from build123d import *

# Parameters (mm, degrees)
SKETCH1_R             = 0.6
BOSS_EXTRUDE1_DEPTH   = 1
SKETCH1_W             = 37.4
SKETCH1_H             = 2.5
BOSS_EXTRUDE1_2_DEPTH = 1
BOSS_EXTRUDE1_3_DEPTH = 1
BOSS_EXTRUDE1_4_DEPTH = 1
SKETCH1_W_2           = 9.2
BOSS_EXTRUDE1_5_DEPTH = 1
BOSS_EXTRUDE2_DEPTH   = 1.5
SKETCH4_W             = 3.5
SKETCH4_H             = 2.5
BOSS_EXTRUDE3_DEPTH   = 3.8
FILLET1_R             = 0.4


with BuildPart() as part:
    # Sketch1 → Boss-Extrude1 (new body)
    with BuildSketch(Plane(origin=(0, 0, 0), x_dir=(1, 0, 0), z_dir=(0, 1, 0))):
        Polygon((-22.2, 30), (-25.229966902, 30), (-40, 30), (-40, 0), (-25.229966902, 0), (-22.2, 0), (-22.2, 2.5), (-37.5, 2.5), (-37.5, 27.5), (-22.2, 27.5), align=None)
        with Locations((-38.75, 1.25)):
            Circle(SKETCH1_R, mode=Mode.SUBTRACT)
        with Locations((-38.75, 28.75)):
            Circle(SKETCH1_R, mode=Mode.SUBTRACT)
    extrude(amount=-BOSS_EXTRUDE1_DEPTH)



with BuildPart() as body_2:
    # Sketch1 → Boss-Extrude1 2 (new body)
    with BuildSketch(Plane(origin=(0, 0, 0), x_dir=(1, 0, 0), z_dir=(0, 1, 0))):
        with Locations((0, 1.25)):
            Rectangle(SKETCH1_W, SKETCH1_H)
    extrude(amount=-BOSS_EXTRUDE1_2_DEPTH)


with BuildPart() as body_3:
    # Sketch1 → Boss-Extrude1 3 (new body)
    with BuildSketch(Plane(origin=(0, 0, 0), x_dir=(1, 0, 0), z_dir=(0, 1, 0))):
        Polygon((12, 30), (10, 30), (9.5, 30), (9.5, 27.5), (18.7, 27.5), (18.7, 30), align=None)
    extrude(amount=-BOSS_EXTRUDE1_3_DEPTH)


with BuildPart() as body_4:
    # Sketch1 → Boss-Extrude1 4 (new body)
    with BuildSketch(Plane(origin=(0, 0, 0), x_dir=(1, 0, 0), z_dir=(0, 1, 0))):
        Polygon((25.229966902, 30), (22.2, 30), (22.2, 27.5), (37.5, 27.5), (37.5, 2.5), (22.2, 2.5), (22.2, 0), (25.229966902, 0), (40, 0), (40, 30), align=None)
        with Locations((38.75, 1.25)):
            Circle(SKETCH1_R, mode=Mode.SUBTRACT)
        with Locations((38.75, 28.75)):
            Circle(SKETCH1_R, mode=Mode.SUBTRACT)
    extrude(amount=-BOSS_EXTRUDE1_4_DEPTH)


with BuildPart() as body_5:
    # Sketch1 → Boss-Extrude1 5 (new body)
    with BuildSketch(Plane(origin=(0, 0, 0), x_dir=(1, 0, 0), z_dir=(0, 1, 0))):
        with Locations((-14.1, 28.75)):
            Rectangle(SKETCH1_W_2, SKETCH1_H)
    extrude(amount=-BOSS_EXTRUDE1_5_DEPTH)


with BuildPart() as part_1:
    add(part.part)

    add(body_2.part)  # Boss-Extrude2 merges body 2

    add(body_3.part)  # Boss-Extrude2 merges body 3

    add(body_4.part)  # Boss-Extrude2 merges body 4

    add(body_5.part)  # Boss-Extrude2 merges body 5
    # Sketch3 → Boss-Extrude2 (add)
    with BuildSketch(Plane(origin=(0, 0, 0), x_dir=(1, 0, 0), z_dir=(0, 1, 0))):
        Polygon((-22.2, 27.5), (-37.5, 27.5), (-37.5, 2.5), (-22.2, 2.5), (-22.2, 0), (-18.7, 0), (-18.7, 2.5), (-9.5, 2.5), (-9.5, 27.5), (-18.7, 27.5), (-18.7, 30), (-22.2, 30), align=None)
        Polygon((9.5, 27.5), (18.7, 27.5), (18.7, 30), (22.2, 30), (22.2, 27.5), (37.5, 27.5), (37.5, 2.5), (22.2, 2.5), (22.2, 0), (18.7, 0), (18.7, 2.5), (9.5, 2.5), align=None)
    extrude(amount=-BOSS_EXTRUDE2_DEPTH)

    # Sketch4 → Boss-Extrude3 (add)
    with BuildSketch(Plane(origin=(0, 0, 0), x_dir=(1, 0, 0), z_dir=(0, 1, 0))):
        with Locations((-20.45, 28.75)):
            Rectangle(SKETCH4_W, SKETCH4_H)
        with Locations((20.45, 28.75)):
            Rectangle(SKETCH4_W, SKETCH4_H)
        with Locations((-20.45, 1.25)):
            Rectangle(SKETCH4_W, SKETCH4_H)
        with Locations((20.45, 1.25)):
            Rectangle(SKETCH4_W, SKETCH4_H)
    extrude(amount=-BOSS_EXTRUDE3_DEPTH)

    # Fillet1
    fillet1_edges = [part_1.edges().sort_by_distance(p)[0] for p in [
        (-22.2, -2.65, -27.5),
        (-18.7, -2.65, -27.5),
        (-18.7, -2.4, -30),
        (-22.2, -2.4, -30),
        (14.1, -1, -30),
        (18.7, -2.4, -30),
        (20.45, -3.8, -30),
        (22.2, -2.4, -30),
        (31.1, -1, -30),
        (40, -0.5, -30),
        (24.75, 0, -30),
        (9.5, -0.5, -30),
        (-18.7, -2.4, 0),
        (-20.45, -3.8, 0),
        (-22.2, -2.4, 0),
        (-31.1, -1, 0),
        (-40, -0.5, 0),
        (0, 0, 0),
        (40, -0.5, 0),
        (31.1, -1, 0),
        (22.2, -2.4, 0),
        (20.45, -3.8, 0),
        (18.7, -2.4, 0),
        (0, -1, 0),
        (-40, -1, -15),
        (0, -1, -2.5),
        (9.5, -1.5, -15),
        (-9.5, -1.5, -15),
        (40, -1, -15),
        (37.5, -1.5, -15),
        (-37.5, -1.5, -15),
        (-18.7, -2.65, -2.5),
        (-22.2, -2.65, -2.5),
        (18.7, -2.65, -2.5),
        (22.2, -2.65, -2.5),
        (22.2, -2.65, -27.5),
        (18.7, -2.65, -27.5),
    ]]
    fillet(fillet1_edges, radius=FILLET1_R)


solid = part_1.part
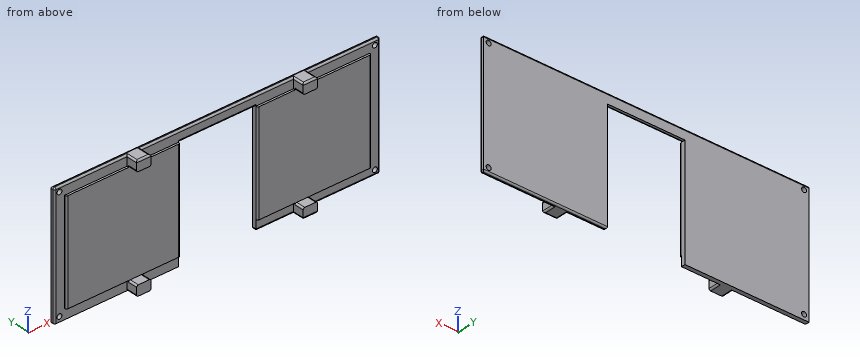
Check sheet for the modelled part. Datum: model origin and axes. Units: mm. Round coordinates to 2 decimals unless told otherwise and drop trailing zeros. Loops run counter-clockwise (first coordinate to the right, second up) from the corner with the lowest first, then second, coordinate; pieces in that order, holes last. Notation, with made-up numbers: M 67.5,-5.75 L 73.5,-5.75 A19 cw 73.5,23.25 Z; hole C 82.25,12.25 d11. An arc over 180 degrees is marked long. One line per question, with ' | ' between items. Start each with the question number.
Item 1: Section check D-D (x = -30). Record the boundary of the cut face in (y, z), and give its area (3 significant figures).
Item 2: Section check C-C (x = 21). Record the boundary of the cut face in (y, z), and give its area (3 significant figures).
Item 3: Gauge pin test, flat ends, axial feed: pin 1 Ø0.6 at (x, y) = (32.5, -1.5) entering from -Z; pin 2 Ø1.6 at (x, z) = (38.75, -28.75) entering from -Y; pin 3 Ø0.5 at (x, y) = (1.5, 0) entering from -Z; pin 4 Ø0.7 at (x, z) = (-38.75, -1.25) entering from -Y. Record the tip position at first contact, or that the pin passes through.
Item 4: Scan lines: probe 1 along Z at (x, y) = (-38.75, -0.35); probe 2 along X at (y, z) = (-0.2, -1.25); probe 3 along X at (y, z) = (-0.7, -28.75). Record each from-to range of solid material in increasing order.
Item 5: Section check A-A (z = -18.5). Record the boundary of the cut face in (x, y), and give its area (3 significant figures).
Item 6: Section check B-B (y = -2.1). State how many separate pieces and enclosed holes the cut face has, and give its area (3 significant figures).
Worked out:
1) outline: M -1.5,-27.5 L -1,-27.5 L -1,-30 L 0,-30 L 0,-0.4 A0.4 ccw -0.4,0 L -0.6,0 A0.4 ccw -1,-0.4 L -1,-2.5 L -1.5,-2.5 Z | area: 42.4 mm^2
2) outline: M -3.8,-29.6 A0.4 ccw -3.4,-30 L -0.4,-30 A0.4 ccw 0,-29.6 L 0,-0.4 A0.4 ccw -0.4,0 L -3.4,0 A0.4 ccw -3.8,-0.4 L -3.8,-2.5 L -1.5,-2.5 L -1.5,-27.5 L -3.8,-27.5 Z | area: 56.4 mm^2
3) pin 1: z = -27.5 | pin 2: y = -1 | pin 3: z = -2.5 | pin 4: through
4) probe 1: -30 to -29.35, -28.15 to -1.85, -0.65 to 0 | probe 2: -40 to -39.35, -38.15 to 38.15, 39.35 to 40 | probe 3: -39.99 to -39.35, -38.15 to -9.5, 9.5 to 38.15, 39.35 to 39.99
5) outline: M -40,-0.6 A0.4 ccw -39.6,-1 L -37.5,-1 L -37.5,-1.1 A0.4 ccw -37.1,-1.5 L -9.9,-1.5 A0.4 ccw -9.5,-1.1 L -9.5,0 L -40,0 Z; M 9.5,-1.1 A0.4 ccw 9.9,-1.5 L 37.1,-1.5 A0.4 ccw 37.5,-1.1 L 37.5,-1 L 39.6,-1 A0.4 ccw 40,-0.6 L 40,0 L 9.5,0 Z | area: 88.8 mm^2
6) separate pieces: 4 | enclosed holes: 0 | area: 34.5 mm^2
